Build history of the part. All positions in model axes, mm. A direction names the side the tool comes from. Round coordinates to 2 decimals unless told otherwise and drop trailing zeros. Write each loop counter-clockwise with the first axis right and the second up, starting at its lowest first coordinate (ties: lowest second). Pieces come first, ordered by that corner, then holes. Notation, with made-up numbers: M 28,85 L 49,85 A20 cw 49,91 Z; hole C -12.5,82 d4. An arc over 180 degrees is marked long. Use a Markdown table: item, result.
Autodesk Inventor part; units mm, degrees
ref_plane "YZ Plane" through (0, 0, 0) normal (1, 0, 0) x (0, 1, 0)
ref_plane "XZ Plane" through (0, 0, 0) normal (0, 1, 0) x (-1, 0, 0)
ref_plane "XY Plane" through (0, 0, 0) normal (0, 0, 1) x (1, 0, 0)
sketch "Sketch1" plane through (0, 0, 0) normal (1, 0, 0) x (0, 1, 0)
  line L0 (0, 0) -> (45, 0)
  line L1 (45, 0) -> (45, -30)
  line L2 (45, -30) -> (0, -30)
  line L3 (0, -30) -> (0, 0)
  dimension "d0" = 45
  dimension "d1" = 30
extrude "Extrusion1" add sketch "Sketch1" along normal blind 3
sketch "Sketch2" plane through (3, 0, 0) normal (1, 0, 0) x (0, 0, -1)
  line L0 (30, 45) -> (0, 45)
  line L1 (6, 45) -> (12, 45)
  line L2 (12, 45) -> (12, 42)
  line L3 (6, 42) -> (6, 45)
  line L4 (0, 45) -> (0, 0)
  line L5 (18, 45) -> (24, 45)
  line L6 (24, 45) -> (24, 42)
  line L7 (18, 42) -> (18, 45)
  line L8 (30, 0) -> (30, 45)
  line L9 (6, 42) -> (7.4, 42)
  line L10 (7.4, 42) -> (7.4, 34.2)
  line L11 (7.4, 34.2) -> (6.2, 34.2)
  line L12 (6.2, 34.2) -> (6.2, 31.45)
  line L13 (6.2, 31.45) -> (7.4, 31.45)
  line L14 (7.4, 31.45) -> (7.4, 24.8)
  line L15 (7.4, 24.8) -> (10.6, 24.8)
  line L16 (10.6, 24.8) -> (10.6, 31.45)
  line L17 (10.6, 31.45) -> (11.8, 31.45)
  line L18 (11.8, 31.45) -> (11.8, 34.2)
  line L19 (11.8, 34.2) -> (10.6, 34.2)
  line L20 (10.6, 42) -> (12, 42)
  line L21 (10.6, 34.2) -> (10.6, 42)
  line L22 (18, 42) -> (19.4, 42)
  line L23 (19.4, 42) -> (19.4, 34.2)
  line L24 (19.4, 34.2) -> (18.2, 34.2)
  line L25 (18.2, 34.2) -> (18.2, 31.45)
  line L26 (18.2, 31.45) -> (19.4, 31.45)
  line L27 (19.4, 24.8) -> (19.4, 31.45)
  line L28 (19.4, 24.8) -> (22.6, 24.8)
  line L29 (22.6, 24.8) -> (22.6, 31.45)
  line L30 (22.6, 31.45) -> (23.8, 31.45)
  line L31 (23.8, 31.45) -> (23.8, 34.2)
  line L32 (23.8, 34.2) -> (22.6, 34.2)
  line L33 (22.6, 42) -> (24, 42)
  line L34 (22.6, 42) -> (22.6, 34.2)
  dimension "d4" = 6
  dimension "d6" = 6
  dimension "d18" = 6
  dimension "d19" = 3
  dimension "d20" = 6
  dimension "d21" = 6
  dimension "d22" = 1.4
  dimension "d23" = 7.8
  dimension "d24" = 1.2
  dimension "d25" = 2.75
  dimension "d26" = 1.2
  dimension "d27" = 6.65
  dimension "d28" = 3.2
  dimension "d29" = 1.2
  dimension "d30" = 1.4
  dimension "d31" = 1.2
  dimension "d32" = 3.2
  dimension "d33" = 1.2
  dimension "d34" = 20.2
extrude "Extrusion2" cut sketch "Sketch2" against normal blind 4
fillet "Fillet1" radius 7 2 edges at (1.5, 0, 0) (1.5, 0, -30)
sketch "Sketch3" plane through (3, 0, 0) normal (1, 0, 0) x (0, 0, -1)
  circle A0 centre (15, 12) radius 1.5
  line L0 (0, 45) -> (0, 7)
  line L1 (7, 0) -> (23, 0)
  point P0 (0, 0)
  dimension "d10" = 3
  dimension "d11" = 15
  dimension "d12" = 12
extrude "Extrusion3" cut sketch "Sketch3" against normal blind 4
properties part number "axel mount (3mm shaft)" material "Plywood, Finish"
Q1. Drop flat-ended pins along their axis: P1, Ø0.7, axis at x = 1, z = -11.5, coming from the +Y side; P2, Ø1.5, axis at x = 1.5, z = -9, coming from the +Y side. Give the stop position or say it passes through.
Response values:
| item | result |
|---|---|
| P1 | stops at y = 42 |
| P2 | stops at y = 24.8 |
Q2. Two-plate mould, pull along Y, no slides. Class faces 1 (the flat face through (2, 34.2, -11)), 2 (the flat face through (2, 28, -19.4)), 3 (the flat face through (1, 45, -3)): +Y half, -Y half, draft (parallel to the pull), parting line (faces both ways), or undercut.
Response values:
| item | result |
|---|---|
| face 1 | undercut |
| face 2 | draft |
| face 3 | +Y half |
Q3. Which spindle directions (+Z, -Z, +X, -X, +Y, -Y) get a long thin tool onto all of the face, cutting with end or side? Do faces 4 (the flat face through (2, 31.45, -7)), 5 (the flat face through (3, 22, -15)), 6 (the flat face through (2, 42, -7)). Say none if no direction does.
Response values:
| item | result |
|---|---|
| face 4 | +X, -X |
| face 5 | +Z, -Z, +X, +Y, -Y |
| face 6 | +X, -X, +Y |
Q4. Drill centre lines: L1, parallel to Z at x = 0.85, y = 43.5; L2, parallel to Z at x = 2.55, y = 40; L3, parallel to Y at x = 1.75, z = -9.5. Where is each one in solid material? Low to high.
Response values:
| item | result |
|---|---|
| L1 | z = -30 to -24, -18 to -12, -6 to 0 |
| L2 | z = -30 to -22.6, -19.4 to -10.6, -7.4 to 0 |
| L3 | y = 0 to 24.8 |
Q5. Cut at A-A on z = -15. Give the cut face in (x, y), and give its area (3 significant figures).
Response values:
| item | result |
|---|---|
| outline | M 0,0 L 3,0 L 3,10.5 L 0,10.5 Z; M 0,13.5 L 3,13.5 L 3,45 L 0,45 Z |
| area | 126 mm2 |
Q6. Cut at B-B on y = 12. Give the cut face in (x, z), and give its area (3 significant figures).
Response values:
| item | result |
|---|---|
| outline | M 0,-30 L 3,-30 L 3,-16.5 L 0,-16.5 Z; M 0,-13.5 L 3,-13.5 L 3,0 L 0,0 Z |
| area | 81.0 mm2 |
